Geometry: final body of the model. Coordinates: model frame, mm. A direction names the side the tool comes from. Coordinates: 2 decimals unless noted, no trailing zeros. Write each loop counter-clockwise with the first axis right and the second up, starting at its lowest first coordinate (ties: lowest second). Pieces come first, ordered by that corner, then holes. Notation, with made-up numbers: (78, -1) - (89, -1) arc R16 ccw to (89, 4) - close; hole circle Ø5 at (44, -7). An arc over 180 degrees is marked (long way). Put each result on its own line as item: value.
```python
from build123d import *

# Parameters (mm, degrees)
BOSS_EXTRUDE1_DEPTH     = 9.5
FILLET5_R               = 5
CUT_EXTRUDE1_DEPTH      = 30.898829409
CUT_EXTRUDE1_DEPTH_BACK = 30.898829409
SKETCH2_R               = 3.175
FILLET1_R               = 5


with BuildPart() as part:
    # Sketch1 → Boss-Extrude1 (new body)
    with BuildSketch(Plane.XY):
        with BuildLine():
            Line((11.5, 0), (26, 0))
            Line((26, 0), (26, 4))
            Line((26, 4), (14.76787053, 4))
            ThreePointArc((14.76787053, 4), (0, 15.3), (-14.76787053, 4))
            Line((-14.76787053, 4), (-26, 4))
            Line((-26, 4), (-26, 0))
            Line((-26, 0), (-11.5, 0))
            ThreePointArc((-11.5, 0), (0, 11.5), (11.5, 0))
        make_face()
    extrude(amount=BOSS_EXTRUDE1_DEPTH)

    # Fillet5
    fillet5_edges = [part.edges().sort_by_distance(p)[0] for p in [
        (-14.76787053, 4, 4.75),
        (14.76787053, 4, 4.75),
    ]]
    fillet(fillet5_edges, radius=FILLET5_R)

    # Sketch2 → Cut-Extrude1 (cut, two sides: drawn at the far end of the back side and taken through both)
    with BuildSketch(Plane(origin=(0, 4, 0), x_dir=(1, 0, 0), z_dir=(0, 1, 0)).offset(-CUT_EXTRUDE1_DEPTH_BACK)):
        with Locations(Location((-21, -4.75, 0), (0, 0, 270))):
            Circle(SKETCH2_R)
        with Locations(Location((21, -4.75, 0), (0, 0, 270))):
            Circle(SKETCH2_R)
    extrude(amount=CUT_EXTRUDE1_DEPTH + CUT_EXTRUDE1_DEPTH_BACK, mode=Mode.SUBTRACT)

    # Fillet1
    # the kernel refuses this fillet: 5 mm, written as the material it takes off along each edge
    with BuildSketch(Plane(origin=(-26, 16.5, 0), x_dir=(1, 0, 0), z_dir=(0, -1, 0))) as fillet1_piece_1:
        with BuildLine():
            CenterArc((FILLET1_R, FILLET1_R), FILLET1_R, 180, 90)
            Line((0, FILLET1_R), (0, 0))
            Line((0, 0), (FILLET1_R, 0))
        make_face()
    extrude(amount=29, mode=Mode.SUBTRACT)
    with BuildSketch(Plane(origin=(26, -12.5, 0), x_dir=(0, 0, 1), z_dir=(0, 1, 0)), Plane(origin=(26, -12.5, 9.5), x_dir=(-1, 0, 0), z_dir=(0, 1, 0)), Plane(origin=(-26, 16.5, 9.5), x_dir=(1, 0, 0), z_dir=(0, -1, 0))) as fillet1_piece_2:
        with BuildLine():
            CenterArc((FILLET1_R, -FILLET1_R), FILLET1_R, 90, 90)
            Line((0, -FILLET1_R), (0, 0))
            Line((0, 0), (FILLET1_R, 0))
        make_face()
    extrude(amount=29, mode=Mode.SUBTRACT)


solid = part.part
```
1. Section query A-A (y = 2). Return loops of the section in (x, z) (3 decimals).
Answer below:
outline: (-25.994, 4.75) arc R5 ccw to (-21, 0) - (-11.325, 0) - (-11.325, 9.5) - (-21, 9.5) arc R5 ccw to start; (11.325, 0) - (21, 0) arc R5 ccw to (25.994, 4.75) arc R5 ccw to (21, 9.5) - (11.325, 9.5) - close; hole circle Ø6.35 at (-21, 4.75); hole circle Ø6.35 at (21, 4.75)
2. Section query D-D (x = 0). Return loops of the section in (y, z).
Answer below:
outline: (11.5, 0) - (15.3, 0) - (15.3, 9.5) - (11.5, 9.5) - close
3. Section query C-C (y = 9). Return loops of the section in (x, z), then the cut area to 3 significant figures.
Answer below:
outline: (-12.37, 0) - (-7.16, 0) - (-7.16, 9.5) - (-12.37, 9.5) - close; (7.16, 0) - (12.37, 0) - (12.37, 9.5) - (7.16, 9.5) - close
area: 99.1 mm²
4. Mould query, pull axis X, two halves, no side actions, for faces 1 (the cylindrical face through (-24, 2, 1)), 2 (the flat face through (-25, 4, 5)), 3 (the cylindrical face through (-17.85, 1.98, 4.34)). Classes: +X half, -X half, draft (parallel to the pull), parting line (faces both ways), or undercut.
Answer below:
face 1: -X half
face 2: draft
face 3: undercut
5. Set-up query: faces 4 (the flat face through (24, 4, 3)), 5 (the cylindrical face through (17.9, 1.98, 4.06)). Return all of +Z, -Z, +X, -X, +Y, -Y with unobstructed straight access to the full face (end or side cutting, diameter ignored); none if empty.
Answer below:
face 4: +Z, -Z, +X, +Y
face 5: +Y, -Y
6. Pin query (flat end, axial travel): pin 1 Ø1.5 at (y, z) = (13.5, 5.5) entering from -X; pin 2 Ø3 at (x, z) = (-8.5, 4.5) entering from +Y; pin 3 Ø3 at (y, z) = (5, 6) entering from +X. Return the tip coordinate at first contact, or that it passes through.
Answer below:
pin 1: stops at x = -8.46
pin 2: stops at y = 13.6
pin 3: stops at x = 25.99
7. Ray query, probe 1 along Z at (x, y) = (-21, 2.5) (3 decimals); probe 2 along X at (y, z) = (3.05, 4.75) (3 decimals); probe 3 along X at (y, z) = (2.6, 4.75) (3 decimals). Return the intervals inside material, ascending. Write a range as from..to.
Answer below:
probe 1: z = 0..1.575, 7.925..9.5
probe 2: x = -25.994..-24.175, -17.825..-11.088, 11.088..17.825, 24.175..25.994
probe 3: x = -25.994..-24.175, -17.825..-11.202, 11.202..17.825, 24.175..25.994
8. Section query B-B (z = 2.5). Return loops of the section in (x, y).
Answer below:
outline: (-25.33, 0) - (-23.24, 0) - (-23.24, 4) - (-25.33, 4) - close; (-18.76, 0) - (-11.5, 0) arc R11.5 cw to (11.5, 0) - (18.76, 0) - (18.76, 4) - (18.2, 4) arc R5 cw to (13.71, 6.78) arc R15.3 ccw to (-13.71, 6.78) arc R5 cw to (-18.2, 4) - (-18.76, 4) - close; (23.24, 0) - (25.33, 0) - (25.33, 4) - (23.24, 4) - close
